Geometry: final body of the model. Coordinates: model frame, mm. Give positions to 0.01 mm unless a question says otherwise; leave off trailing zeros. Write each loop counter-clockwise with the first axis right and the second up, starting at its lowest first coordinate (ties: lowest second). Pieces come first, ordered by that corner, then holes.
Q1. Section B-B (x = 0). Return the cut outline in (y, z).
Q2. Section C-C (z = 0). Return the cut outline in (x, y) (3 decimals), plus the area to 3 significant figures.
Q3. Pin query (flat end, axial travel): pin 1 Ø1 at (y, z) = (2, 31) entering from -X; pin 2 Ø0.9 at (x, y) = (59, 2) entering from -Z. Return the tip coordinate at first contact, or that it passes through.
Q4. Section A-A (z = -45). Return the cut outline in (x, y).
Q5. Line query: line 1 (X direction, y = 2.2, z = -63); line 2 (Z direction, x = -13, y = 0.8); line 3 (X direction, y = 1.95, z = -22). Output: solid intervals per line, ascending.
Q6. Section D-D (z = -60). Return the cut outline in (x, y), plus the area to 3 significant figures.
from build123d import *

# Parameters (mm, degrees)
SKETCH1_R           = 75
BOSS_EXTRUDE1_DEPTH = 3
SKETCH2_W           = 10
SKETCH2_H           = 45
CUT_EXTRUDE1_DEPTH  = 6.35
SKETCH3_R           = 7.75
CUT_EXTRUDE2_DEPTH  = 10
CUT_EXTRUDE3_DEPTH  = 10
FILLET2_R           = 10
SKETCH7_R           = 3
CUT_EXTRUDE5_DEPTH  = 3
CUT_EXTRUDE6_DEPTH  = 3
SKETCH8_R           = 1.7145
CUT_EXTRUDE7_DEPTH  = 10


with BuildPart() as part:
    # Sketch1 → Boss-Extrude1 (new body)
    with BuildSketch(Plane(origin=(0, 0, 0), x_dir=(1, 0, 0), z_dir=(0, 1, 0))):
        Circle(SKETCH1_R)
    extrude(amount=BOSS_EXTRUDE1_DEPTH)

    # Sketch2 → Cut-Extrude1 (cut)
    with BuildSketch(Plane(origin=(0, 3, 0), x_dir=(1, 0, 0), z_dir=(0, 1, 0))):
        with Locations((-61, 0)):
            Rectangle(SKETCH2_W, SKETCH2_H)
        with Locations((61, 0)):
            Rectangle(SKETCH2_W, SKETCH2_H)
    extrude(amount=-CUT_EXTRUDE1_DEPTH, mode=Mode.SUBTRACT)

    # Sketch3 → Cut-Extrude2 (cut)
    with BuildSketch(Plane(origin=(0, 3, 0), x_dir=(1, 0, 0), z_dir=(0, 1, 0))):
        with Locations((0, -25)):
            Circle(SKETCH3_R)
        with Locations((0, 60)):
            Circle(SKETCH3_R)
    extrude(amount=-CUT_EXTRUDE2_DEPTH, mode=Mode.SUBTRACT)

    # Sketch4 → Cut-Extrude3 (cut)
    with BuildSketch(Plane(origin=(0, 3, 0), x_dir=(1, 0, 0), z_dir=(0, 1, 0))):
        with BuildLine():
            ThreePointArc((-33.160552015, -67.270928268), (0, -47.932265908), (33.160552015, -67.270928268))
            ThreePointArc((33.160552015, -67.270928268), (0, -75), (-33.160552015, -67.270928268))
        make_face()
    extrude(amount=-CUT_EXTRUDE3_DEPTH, mode=Mode.SUBTRACT)

    # Fillet2
    fillet2_edges = [part.edges().sort_by_distance(p)[0] for p in [
        (-33.160552015, 1.5, 67.270928268),
        (33.160552015, 1.5, 67.270928268),
    ]]
    fillet(fillet2_edges, radius=FILLET2_R)

    # Sketch7 → Cut-Extrude5 (cut)
    with BuildSketch(Plane(origin=(0, 3, 0), x_dir=(1, 0, 0), z_dir=(0, 1, 0))):
        with Locations((-48.975, 0)):
            Circle(SKETCH7_R)
        with Locations((-17.225, -7.9375)):
            Circle(SKETCH7_R)
        with Locations((-17.225, 7.9375)):
            Circle(SKETCH7_R)
        with Locations((17.225, 7.9375)):
            Circle(SKETCH7_R)
        with Locations((17.225, -7.9375)):
            Circle(SKETCH7_R)
        with Locations((48.975, 0)):
            Circle(SKETCH7_R)
    extrude(amount=-CUT_EXTRUDE5_DEPTH, mode=Mode.SUBTRACT)

    # Sketch6 → Cut-Extrude6 (cut)
    with BuildSketch(Plane(origin=(0, 3, 0), x_dir=(1, 0, 0), z_dir=(0, 1, 0))):
        Polygon((-15, 64.502061929), (-18.8989, 62.251030965), (-18.8989, 57.748969035), (-15, 55.497938071), (-11.1011, 57.748969035), (-11.1011, 62.251030965), align=None)
        Polygon((15, 64.502061929), (11.1011, 62.251030965), (11.1011, 57.748969035), (15, 55.497938071), (18.8989, 57.748969035), (18.8989, 62.251030965), align=None)
        Polygon((-15, -20.497938071), (-18.8989, -22.748969035), (-18.8989, -27.251030965), (-15, -29.502061929), (-11.1011, -27.251030965), (-11.1011, -22.748969035), align=None)
        Polygon((15, -20.497938071), (11.1011, -22.748969035), (11.1011, -27.251030965), (15, -29.502061929), (18.8989, -27.251030965), (18.8989, -22.748969035), align=None)
    extrude(amount=-CUT_EXTRUDE6_DEPTH, mode=Mode.SUBTRACT)

    # Sketch8 → Cut-Extrude7 (cut)
    with BuildSketch(Plane(origin=(0, 0, 0), x_dir=(-1, 0, 0), z_dir=(0, -1, 0))):
        with Locations((45, -45)):
            Circle(SKETCH8_R)
        with Locations((-45, -45)):
            Circle(SKETCH8_R)
        with Locations((-45, 45)):
            Circle(SKETCH8_R)
        with Locations((45, 45)):
            Circle(SKETCH8_R)
    extrude(amount=-CUT_EXTRUDE7_DEPTH, mode=Mode.SUBTRACT)


solid = part.part
Computed:
1. outline: (0, -75) - (3, -75) - (3, -67.75) - (0, -67.75) - close; (0, -52.25) - (3, -52.25) - (3, 17.25) - (0, 17.25) - close; (0, 32.75) - (3, 32.75) - (3, 47.93) - (0, 47.93) - close
2. outline: (-75, 0) - (-66, 0) - (-66, 3) - (-75, 3) - close; (-56, 0) - (-51.975, 0) - (-51.975, 3) - (-56, 3) - close; (-45.975, 0) - (45.975, 0) - (45.975, 3) - (-45.975, 3) - close; (51.975, 0) - (56, 0) - (56, 3) - (51.975, 3) - close; (66, 0) - (75, 0) - (75, 3) - (66, 3) - close
2. area: 354 mm2
3. pin 1: stops at x = -68.52
3. pin 2: stops at z = -46.87
4. outline: (-60, 0) - (-46.71, 0) - (-46.71, 3) - (-60, 3) - close; (-43.29, 0) - (43.29, 0) - (43.29, 3) - (-43.29, 3) - close; (46.71, 0) - (60, 0) - (60, 3) - (46.71, 3) - close
5. line 1: x = -40.69 to -17.6, -12.4 to -7.15, 7.15 to 12.4, 17.6 to 40.69
5. line 2: z = -73.86 to -63.35, -56.65 to 21.65, 28.35 to 50.22
5. line 3: x = -71.7 to -66, -56 to 56, 66 to 71.7
6. outline: (-45, 0) - (-18.9, 0) - (-18.9, 3) - (-45, 3) - close; (-11.1, 0) - (-7.75, 0) - (-7.75, 3) - (-11.1, 3) - close; (7.75, 0) - (11.1, 0) - (11.1, 3) - (7.75, 3) - close; (18.9, 0) - (45, 0) - (45, 3) - (18.9, 3) - close
6. area: 177 mm2
